```python
from build123d import *

# Parameters (mm, degrees)
SKETCH1_W           = 11
SKETCH1_H           = 6
OVERMOULD_DEPTH     = 20
SKETCH2_R           = 2.25
STRAIN_RELIEF_DEPTH = 8
LEAD_PROFILE_R      = 1.75


with BuildPart() as part:
    # Sketch1 → Overmould (new body)
    with BuildSketch(Plane(origin=(0, 0, 0), x_dir=(1, 0, 0), z_dir=(0, 1, 0))):
        Rectangle(SKETCH1_W, SKETCH1_H)
    extrude(amount=-OVERMOULD_DEPTH)

    # Sketch2 → Strain_relief (add)
    with BuildSketch(Plane(origin=(0, -20, 0), x_dir=(1, 0, 0), z_dir=(0, 1, 0))):
        with Locations(Location((0, 0, 0), (0, 0, 270))):
            Circle(SKETCH2_R)
    extrude(amount=-STRAIN_RELIEF_DEPTH)

    # Lead: sweep along a path in Sketch3
    with BuildLine(Plane.XY) as lead_path:
        Line((0, -28), (0, -33))
        ThreePointArc((0, -33), (-8.786796564, -54.213203436), (-30, -63))
        Line((-30, -63), (-70, -63))
    # Lead profile (on start of the path) → Lead (sweep)
    with BuildSketch(Plane(origin=(0, -28, 0), x_dir=(0, 0, -1), z_dir=(0, -1, 0))):
        Circle(LEAD_PROFILE_R)
    sweep(path=lead_path.line)


solid = part.part
```
The listing builds one solid part. Answer for the finished solid, in the listing's coordinates (mm). A direction names the side the tool comes from. Round coordinates to 2 decimals unless told otherwise and drop trailing zeros. Write each loop counter-clockwise with the first axis right and the second up, starting at its lowest first coordinate (ties: lowest second). Pieces come first, ordered by that corner, then holes. Notation, with made-up numbers: (78.5, 82.25) -> (82.5, 82.25) arc R23 ccw to (82.5, 91.25) -> close; hole circle Ø11 at (-29.75, 39). An arc over 180 degrees is marked (long way). Answer as a JSON object with one key per item and string values. Group by question number.
Q1. Section A-A (z = 0) is taken. Write down the section's boundary in (x, y), plus the area to 3 significant figures.
Q2. Which of the six approach directions +Z, -Z, +X, -X, +Y, -Y give full straight-line access (tool end or side, diameter ignored) to faces 1 (the face through (5.5, -10, 0)), 2 (the face through (-5.5, -10, 0)), 3 (the face through (-2, -28, 0))?
Q3. Section D-D (y = -8) is taken. Write down the section's boundary in (x, z), plus the area to 3 significant figures.
Q4. Straight lines are drawn through the part: line 1 along X through (y, z) = (-12, -1.15); line 2 along Y through (x, z) = (-1.5, -2.5); line 3 along Y through (x, z) = (-8, 0.4). For each, find the intervals that lie inside material, in ascending order.
Q5. Determine the mould class of faces 4 (the face through (0, -10, -3)), 5 (the face through (0, 0, 0)), 6 (the face through (-50.28, -61.29, 0.38)), 7 (the face through (-0.67, -30.535, -1.617)) for opening direction Y: pulls with the +Y half, pulls with the -Y half, needs draft (parallel to the pull), parting line crosses it, or undercut.
Q6. Section C-C (x = -47.5) is taken. Write down the section's boundary in (y, z), plus the area to 3 significant figures.
Q7. Each of these flat-tipped pins is pushed along its axis until it touches: pin 1 Ø3 at (y, z) = (-41, 0) entering from -X; pin 2 Ø2 at (y, z) = (-10, -1.5) entering from -X; pin 3 Ø1.8 at (x, z) = (-1, 0) entering from -Y. Where does it stop, or does it pass through?
Q8. Section B-B (y = -25) is taken. Write down the section's boundary in (x, z).
Check values:
{
 "1": {"outline": "(-70, -64.75) -> (-30, -64.75) arc R31.75 ccw to (1.75, -33) -> (1.75, -28) -> (2.25, -28) -> (2.25, -20) -> (5.5, -20) -> (5.5, 0) -> (-5.5, 0) -> (-5.5, -20) -> (-2.25, -20) -> (-2.25, -28) -> (-1.75, -28) -> (-1.75, -33) arc R28.25 cw to (-30, -61.25) -> (-70, -61.25) -> close", "area": "578 mm^2"},
 "2": {"face 1": "+Z, -Z, +X, +Y, -Y", "face 2": "+Z, -Z, -X, +Y", "face 3": "none"},
 "3": {"outline": "(-5.5, -3) -> (5.5, -3) -> (5.5, 3) -> (-5.5, 3) -> close", "area": "66.0 mm^2"},
 "4": {"line 1": "-5.5 to 5.5", "line 2": "-20 to 0", "line 3": "-55.83 to -50.8"},
 "5": {"face 4": "needs draft", "face 5": "pulls with the +Y half", "face 6": "parting line crosses it", "face 7": "undercut"},
 "6": {"outline": "circle Ø3.5 at (-63, 0)", "area": "9.62 mm^2"},
 "7": {"pin 1": "x = -3.4", "pin 2": "x = -5.5", "pin 3": "y = -47.78"},
 "8": {"outline": "circle Ø4.5 at (0, 0)"}
}
